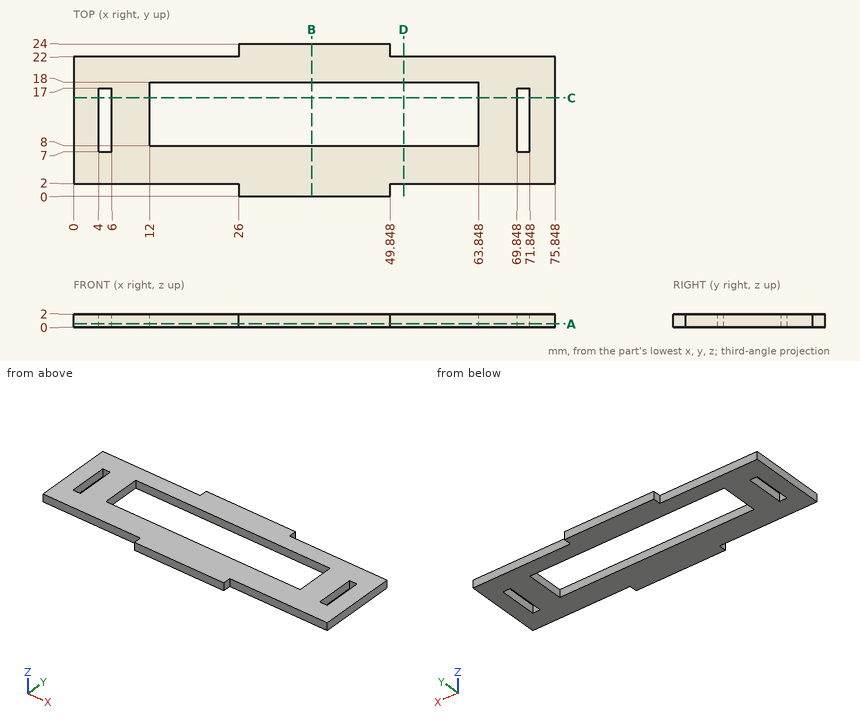
Input: dimensioned drawing with shaded views. Units: mm. Origin: part minimum x, y, z. Coordinates: 2 decimals unless noted, no trailing zeros. Write each loop counter-clockwise with the first axis right and the second up, starting at its lowest first coordinate (ties: lowest second). Pieces come first, ordered by that corner, then holes. Notation, with made-up numbers: M 55.25,-7.75 L 94.25,-7.75 A30 ccw 94.25,14.25 Z; hole C -34,18 d5. An arc over 180 degrees is marked long. Answer as CSV lines item,"result". Start each with the question number.
Q1. Cut plane C-C on y = 15.5. Return the cut outline in (x, z).
Q2. Pin query (flat end, axial travel): P1, Ø0.6, axis at x = 4.5, z = 1, coming from the +Y side; P2, Ø0.6, axis at x = 70.5, z = 1, coming from the -Y side; P3, Ø1, axis at y = 0.5, z = 1.5, coming from the +X side. Return the tip coordinate at first contact, or that it passes through.
Q3. Line query: line 1 (X direction, y = 16, z = 0.45); line 2 (Y direction, x = 29, z = 1.35); line 3 (Y direction, x = 25.5, z = 0.4). Output: solid intervals per line, ascending. Write a range as from..to.
Q4. Cut plane D-D on x = 52. Return the cut outline in (y, z), then the cut area to 3 significant figures.
Q5. Cut plane A-A on z = 0.5. Return the cut outline in (x, y).
Q6. Cut plane B-B on x = 37.5. Return the cut outline in (y, z), then the cut area to 3 significant figures.
Findings below:
1,outline,"M 0,0 L 4,0 L 4,2 L 0,2 Z; M 6,0 L 12,0 L 12,2 L 6,2 Z; M 63.85,0 L 69.85,0 L 69.85,2 L 63.85,2 Z; M 71.85,0 L 75.85,0 L 75.85,2 L 71.85,2 Z"
2,P1,"stops at y = 22"
2,P2,"stops at y = 2"
2,P3,"stops at x = 49.85"
3,line 1,"x = 0..4, 6..12, 63.85..69.85, 71.85..75.85"
3,line 2,"y = 0..8, 18..24"
3,line 3,"y = 2..8, 18..22"
4,outline,"M 2,0 L 8,0 L 8,2 L 2,2 Z; M 18,0 L 22,0 L 22,2 L 18,2 Z"
4,area,"20.0 mm2"
5,outline,"M 0,2 L 26,2 L 26,0 L 49.85,0 L 49.85,2 L 75.85,2 L 75.85,22 L 49.85,22 L 49.85,24 L 26,24 L 26,22 L 0,22 Z; hole M 4,7 L 6,7 L 6,17 L 4,17 Z; hole M 12,8 L 63.85,8 L 63.85,18 L 12,18 Z; hole M 69.85,7 L 71.85,7 L 71.85,17 L 69.85,17 Z"
6,outline,"M 0,0 L 8,0 L 8,2 L 0,2 Z; M 18,0 L 24,0 L 24,2 L 18,2 Z"
6,area,"28.0 mm2"
